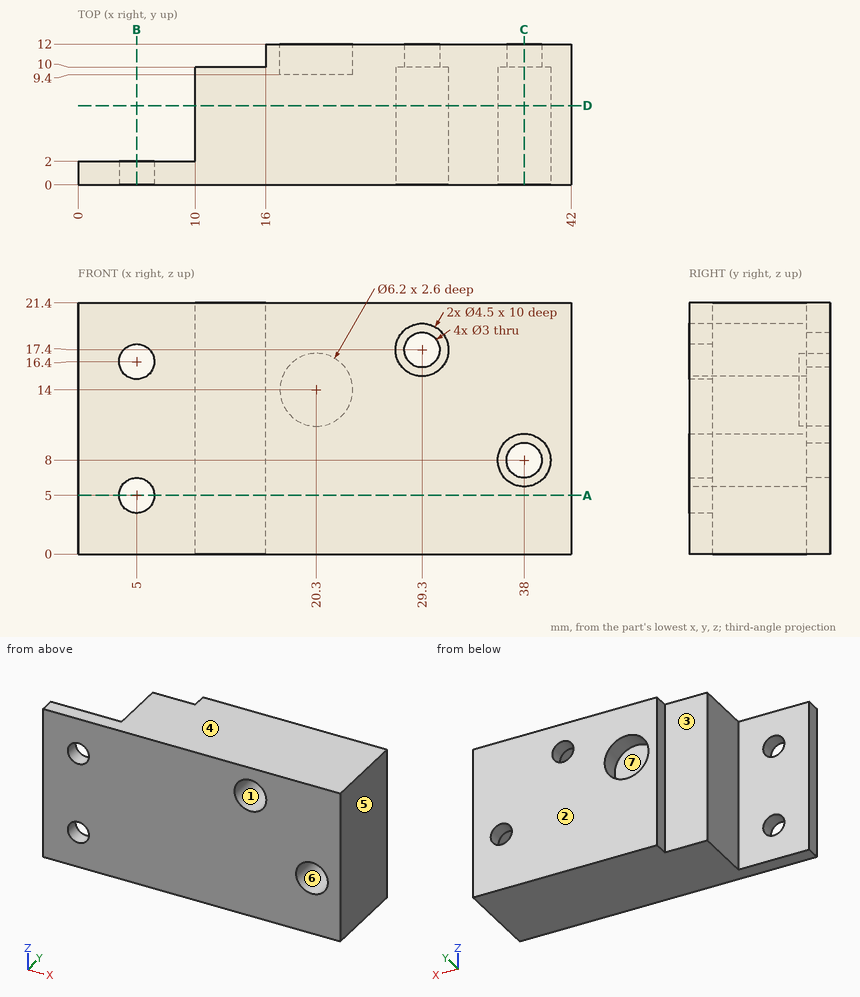
Check sheet for the drawn part. Datum: minimum x, y, z corner. Units: mm. A direction names the side the tool comes from. Give positions to 0.01 mm unless a question says otherwise; leave off trailing zeros. Loops run counter-clockwise (first coordinate to the right, second up) from the corner with the lowest first, then second, coordinate; pieces in that order, holes last. Notation, with made-up numbers: M -39.75,6 L 16.25,6 A31 ccw 16.25,32 Z; hole C 20,42.25 d11. An arc over 180 degrees is marked long. Answer as CSV lines item,"result".
Item 1: Sectioned sample at B-B, the plane x = 5. Enter the section's corners in (y, z).
Reply:
outline,"M 0,0 L 2,0 L 2,3.5 L 0,3.5 Z; M 0,6.5 L 2,6.5 L 2,14.9 L 0,14.9 Z; M 0,17.9 L 2,17.9 L 2,21.4 L 0,21.4 Z"
Item 2: Scan lines: L1, parallel to X at y = 10.5, z = 8; L2, parallel to X at y = 7.25, z = 8; L3, parallel to Y at x = 2, z = 15. Record each from-to range of solid material in increasing order.
Reply:
L1,"16 to 36.5, 39.5 to 42"
L2,"10 to 35.75, 40.25 to 42"
L3,"0 to 2"
Item 3: Depth check by flat-ended pin: pin 1 Ø8 at (x, z) = (7, 6.5) entering from +Y; pin 2 Ø1.9 at (x, z) = (21.5, 13) entering from +Y; pin 3 Ø4 at (y, z) = (5.5, 11.5) entering from -X. Enter the tip coordinate at first touch or a pass-through.
Reply:
pin 1,"y = 10"
pin 2,"y = 9.4"
pin 3,"x = 10"
Item 4: Sectioned sample at D-D, the plane y = 6.75. Enter the section's corners in (x, z).
Reply:
outline,"M 10,0 L 42,0 L 42,21.4 L 10,21.4 Z; hole C 29.3,17.4 d4.5; hole C 38,8 d4.5"
Item 5: Sectioned sample at C-C, the plane x = 38. Enter the section's corners in (y, z).
Reply:
outline,"M 0,0 L 12,0 L 12,6.5 L 10,6.5 L 10,5.75 L 0,5.75 Z; M 0,10.25 L 10,10.25 L 10,9.5 L 12,9.5 L 12,21.4 L 0,21.4 Z"
Item 6: Set-up check for the marked faces 1, 2 and 3: record each of +Z, -Z, +X, -X, +Y, -Y from which the full face is reachable in a straight line by a thin tool's end or side.
Reply:
face 1,"-Y"
face 2,"+Z, -Z, +X, -X, +Y"
face 3,"+Z, -Z, -X, +Y"
Item 7: Draft check along X on the marked faces 4, 5, 6 and 7. Enter one of: pulls with the +X half, pulls with the -X half, needs draft (parallel to the pull), parting line crosses it, or undercut.
Reply:
face 4,"needs draft"
face 5,"pulls with the +X half"
face 6,"undercut"
face 7,"undercut"
Item 8: Sectioned sample at A-A, the plane z = 5. Enter the section's corners in (x, y), then the cut area to 3 significant figures.
Reply:
outline,"M 0,0 L 3.5,0 L 3.5,2 L 0,2 Z; M 6.5,0 L 42,0 L 42,12 L 16,12 L 16,10 L 10,10 L 10,2 L 6.5,2 Z"
area,"386 mm^2"
